```python
from build123d import *

# Parameters (mm, degrees)
SKETCH_1_R          = 1.5
EXTRUDE_1_DEPTH     = 25
SKETCH_2_R          = 2
SKETCH_2_W          = 5
SKETCH_2_H          = 8
CUT_EXTRUDE_1_DEPTH = 29.848743474
CHAMFER_1_SIZE      = 1


with BuildPart() as part:
    # 草图1 → 凸台-拉伸1 (new body)
    with BuildSketch(Plane.XY):
        with BuildLine():
            Line((0, -2.5), (13.5, -2.5))
            Line((13.5, -2.5), (13.5, -1.5))
            Line((13.5, -1.5), (2, -1.5))
            ThreePointArc((2, -1.5), (-1.118033989, 2.236067977), (0, -2.5))
        make_face()
        Circle(SKETCH_1_R, mode=Mode.SUBTRACT)
    extrude(amount=EXTRUDE_1_DEPTH)

    # 草图2 → 切除-拉伸1 (cut, through all)
    with BuildSketch(Plane.XZ.offset(2.5)):
        with Locations(Location((9.25, 20, 0), (0, 0, 270))):
            Circle(SKETCH_2_R)
        with Locations((9.25, 5)):
            Circle(SKETCH_2_R)
        with Locations((0, 4)):
            Rectangle(SKETCH_2_W, SKETCH_2_H)
        with Locations((0, 21)):
            Rectangle(SKETCH_2_W, SKETCH_2_H)
    extrude(amount=-CUT_EXTRUDE_1_DEPTH, mode=Mode.SUBTRACT)

    # 倒角1
    chamfer_1_edges = [part.edges().sort_by_distance(p)[0] for p in [
        (7.25, -1.5, 5),
        (9.25, -1.5, 22),
    ]]
    chamfer(chamfer_1_edges, length=CHAMFER_1_SIZE - 0.0001)  # a hair under: the kernel refuses the full size


solid = part.part
```
Source: CAD feature listing. Evaluate the final solid. Frame: model axes, mm. A direction names the side the tool comes from. Coordinates: 2 decimals unless noted, no trailing zeros. Write each loop counter-clockwise with the first axis right and the second up, starting at its lowest first coordinate (ties: lowest second). Pieces come first, ordered by that corner, then holes. Notation, with made-up numbers: M 70,2.5 L 119,2.5 A13 cw 119,11.5 Z; hole C 26,1 d5. An arc over 180 degrees is marked long. Answer as a JSON object with one key per item and string values.
1. Cut plane A-A on y = 0. Output: boundary loops of the cut face in (x, z).
Evaluation:
{"outline": "M -2.5,8 L -1.5,8 L -1.5,17 L -2.5,17 Z; M 1.5,8 L 2.5,8 L 2.5,17 L 1.5,17 Z"}
2. Access query for faces 1 (the flat face through (2, 0, 17)), 2 (the flat face through (13.5, -2, 12)), 3 (the flat face through (2.5, -2, 4)). Directions: +Z, -Z, +X, -X, +Y, -Y. A direction counts if a zero-diameter tool reaches every point of the face in a straight line with its end or side. Return the directions, or none.
Evaluation:
{"face 1": "+Z, -X, +Y, -Y", "face 2": "+Z, -Z, +X, +Y, -Y", "face 3": "-Z, -X, +Y, -Y"}
3. Ray query, L1, parallel to X at y = 0, z = 10.25; L2, parallel to Y at x = 8, z = 13.75; L3, parallel to Z at x = -1.5, y = 1.75. Return the intervals inside material, ascending.
Evaluation:
{"L1": "-2.5 to -1.5, 1.5 to 2.5", "L2": "-2.5 to -1.5", "L3": "8 to 17"}
4. Cut plane B-B on x = 9.25. State how many separate pieces and enclosed holes the cut face has, plus the area to 3 significant figures.
Evaluation:
{"separate pieces": "3", "enclosed holes": "0", "area": "15.0 mm^2"}
5. Draft query along X for faces 4 (the cylindrical face through (-1.5, 0.07, 12.44)), 5 (the flat face through (2.5, -2, 21)), 6 (the flat face through (2, 0, 8)). Return one class per face: released by +X, released by -X, zero draft, split by the parting line, or undercut.
Evaluation:
{"face 4": "undercut", "face 5": "released by -X", "face 6": "zero draft"}
6. Cut plane D-D on x = -1. Output: boundary loops of the cut face in (y, z), plus the area to 3 significant figures.
Evaluation:
{"outline": "M -2.29,8 L -1.12,8 L -1.12,17 L -2.29,17 Z; M 1.12,8 L 2.29,8 L 2.29,17 L 1.12,17 Z", "area": "21.1 mm^2"}
7. Contact query for flat-ended pins moving along their axis: P1, Ø1.5, axis at y = 0, z = 7, coming from the -X side; P2, Ø9, axis at x = 5, z = 12, coming from the +Y side; P3, Ø1.1, axis at y = -2, z = 5, coming from the -X side; P4, Ø2.5, axis at x = 1, y = -1, coming from the +Z side. Output: stop coordinate, or through.
Evaluation:
{"P1": "through", "P2": "y = 2.45", "P3": "x = 2.5", "P4": "z = 17"}
